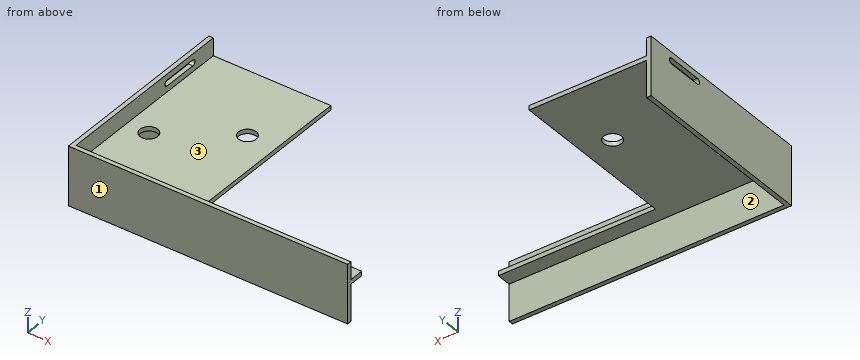
from build123d import *

# Parameters (mm, degrees)
SKETCH1_W           = 80
SKETCH1_H           = 130
BOSS_EXTRUDE1_DEPTH = 3
SKETCH2_R           = 6
CUT_EXTRUDE1_DEPTH  = 153.672852859
SKETCH3_W           = 40
SKETCH3_H           = 130
BOSS_EXTRUDE2_DEPTH = 3
SKETCH4_W           = 190
SKETCH4_H           = 40
BOSS_EXTRUDE3_DEPTH = 3
SKETCH5_W           = 107
SKETCH5_H           = 10
BOSS_EXTRUDE4_DEPTH = 3
CUT_EXTRUDE2_DEPTH  = 230.1156913


with BuildPart() as part:
    # Sketch1 → Boss-Extrude1 (new body)
    with BuildSketch(Plane.XY):
        with Locations((40, 65)):
            Rectangle(SKETCH1_W, SKETCH1_H)
    extrude(amount=BOSS_EXTRUDE1_DEPTH)

    # Sketch2 → Cut-Extrude1 (cut, through all)
    with BuildSketch(Plane.XY.offset(3)):
        with Locations((60, 80)):
            Circle(SKETCH2_R)
        with Locations((15, 50)):
            Circle(SKETCH2_R)
    extrude(amount=-CUT_EXTRUDE1_DEPTH, mode=Mode.SUBTRACT)

    # Sketch3 → Boss-Extrude2 (add)
    with BuildSketch(Plane.ZY):
        with Locations((-5, 65)):
            Rectangle(SKETCH3_W, SKETCH3_H)
    extrude(amount=BOSS_EXTRUDE2_DEPTH)

    # Sketch4 → Boss-Extrude3 (add)
    with BuildSketch(Plane.XZ):
        with Locations((92, -5)):
            Rectangle(SKETCH4_W, SKETCH4_H)
    extrude(amount=-BOSS_EXTRUDE3_DEPTH)

    # Sketch5 → Boss-Extrude4 (add)
    with BuildSketch(Plane(origin=(0, 0, 0), x_dir=(-1, 0, 0), z_dir=(0, 0, -1))):
        with Locations((-133.5, 8)):
            Rectangle(SKETCH5_W, SKETCH5_H)
    extrude(amount=-BOSS_EXTRUDE4_DEPTH)

    # Sketch6 → Cut-Extrude2 (cut, through all)
    with BuildSketch(Plane(origin=(0, 0, 0), x_dir=(0, 0, -1), z_dir=(1, 0, 0))):
        with BuildLine():
            Line((-7.023016919, 111.057268812), (-7.023016919, 87.264774426))
            ThreePointArc((-7.023016919, 87.264774426), (-8.975714476, 85.312076869), (-10.928412033, 87.264774426))
            Line((-10.928412033, 87.264774426), (-10.928412033, 111.057268812))
            ThreePointArc((-10.928412033, 111.057268812), (-8.975714476, 113.00996637), (-7.023016919, 111.057268812))
        make_face()
    extrude(amount=-CUT_EXTRUDE2_DEPTH, mode=Mode.SUBTRACT)


solid = part.part
Verification items for the finished model (mm, model axes). Face numbers are marked on the shaded views. A direction names the side the tool comes from. Round coordinates to 2 decimals unless told otherwise and drop trailing zeros. Loops run counter-clockwise (first coordinate to the right, second up) from the corner with the lowest first, then second, coordinate; pieces in that order, holes last. Notation, with made-up numbers: (-29, 66) - (18, 66) arc R26 ccw to (18, 105) - close; hole circle Ø7 at (-1, 0). An arc over 180 degrees is marked (long way). Use a Markdown table: item, result. Add a question column.
1. Access from +Z, -Z, +X, -X, +Y, -Y to the whole of each face (thin tool, end or side, straight path). Record for the marked faces 1, 2 and 3.
2. Section check D-D, the plane z = -3.5. Record the boundary of the cut face in (x, y).
3. Gauge pin test, flat ends, axial feed: pin 1 (3 mm diameter, centred on x = 165.5, z = -13.5, fed in from +Y); pin 2 (19 mm diameter, centred on x = 60, y = 80, fed in from -Z); pin 3 (1 mm diameter, centred on x = 62.5, y = 35.5, fed in from +Z); pin 4 (1 mm diameter, centred on x = 68.5, z = -1.5, fed in from -Y). Record the tip position at first contact, or that the pin passes through.
4. Thickness scan on probe 1 along Y at (x, z) = (15, 1); probe 2 along Y at (x, z) = (60, 2.4); probe 3 along Y at (x, z) = (116, -13.5). Record the ranges inside material, lowest first. Write a range as [from, to].
5. Section check C-C, the plane x = 37.5. Record the boundary of the cut face in (y, z), plus the area to 3 significant figures.
6. Section check A-A, the plane y = 50. Record the boundary of the cut face in (x, z), plus the area to 3 significant figures.
7. Section check B-B, the plane x = 60. Record the boundary of the cut face in (y, z), plus the area to 3 significant figures.
Checks:
| question | item | result |
|---|---|---|
| 1 | face 1 | +Z, -Z, +X, -X, -Y |
| 1 | face 2 | -Z, +X, +Y |
| 1 | face 3 | +Z, +X, +Y |
| 2 | outline | (-3, 0) - (187, 0) - (187, 3) - (0, 3) - (0, 130) - (-3, 130) - close |
| 3 | pin 1 | stops at y = 3 |
| 3 | pin 2 | stops at z = 0 |
| 3 | pin 3 | stops at z = 3 |
| 3 | pin 4 | stops at y = 0 |
| 4 | probe 1 | y = [0, 44], [56, 130] |
| 4 | probe 2 | y = [0, 74], [86, 130] |
| 4 | probe 3 | y = [0, 3] |
| 5 | outline | (0, -25) - (3, -25) - (3, 0) - (130, 0) - (130, 3) - (3, 3) - (3, 15) - (0, 15) - close |
| 5 | area | 501 mm^2 |
| 6 | outline | (-3, -25) - (0, -25) - (0, 0) - (9, 0) - (9, 3) - (0, 3) - (0, 15) - (-3, 15) - close; (21, 0) - (80, 0) - (80, 3) - (21, 3) - close |
| 6 | area | 324 mm^2 |
| 7 | outline | (0, -25) - (3, -25) - (3, 0) - (74, 0) - (74, 3) - (3, 3) - (3, 15) - (0, 15) - close; (86, 0) - (130, 0) - (130, 3) - (86, 3) - close |
| 7 | area | 465 mm^2 |
